Geometry: final body of the model. Coordinates: model frame, mm. Face numbers are marked on the shaded views. A direction names the side the tool comes from. Round coordinates to 2 decimals unless told otherwise and drop trailing zeros. Write each loop counter-clockwise with the first axis right and the second up, starting at its lowest first coordinate (ties: lowest second). Pieces come first, ordered by that corner, then holes. Notation, with made-up numbers: M -8.75,-6 L 32.25,-6 A24 ccw 32.25,15 Z; hole C 55.25,71 d3. An arc over 180 degrees is marked long. Answer as CSV lines item,"result". Start each with the question number.
Q1. Section query B-B on z = -1. Output: boundary loops of the cut face in (x, y), and give its area (3 significant figures).
Q2. Reachability of the marked faces 1 and 2 from +Z, -Z, +X, -X, +Y, -Y: full face, straight path, thin tool, end or side. Return the list, or none.
Q3. Mould query, pull axis Z, two halves, no side actions, for the marked faces 3, 4, 5 and 6. Classes: pulls with the +Z half, pulls with the -Z half, needs draft (parallel to the pull), parting line crosses it, or undercut.
Q4. Section query C-C on y = -6. Output: boundary loops of the cut face in (x, z).
Q5. Section query A-A on y = -19. Output: boundary loops of the cut face in (x, z), and give its area (3 significant figures).
Q6. Ray query, probe 1 along Y at (x, z) = (24.5, 4.25); probe 2 along Z at (x, y) = (15, -17); probe 3 along Z at (x, y) = (27, -32.5). Return the intervals inside material, ascending.
Q7. First-contact query: pin 1 (2 mm diameter, centred on x = 16, y = -18, fed in from -Z); pin 2 (3 mm diameter, centred on x = 18, z = 16, fed in from -Y); pin 3 (6 mm diameter, centred on x = 5, y = -34, fed in from +Z). Flat tips, straight axial feed; report the tip coordinate or a pass-through.
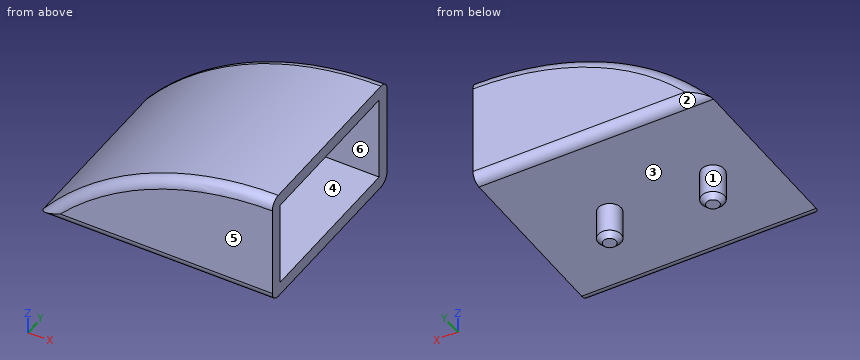
```python
from build123d import *

# Parameters (mm, degrees)
F1_DEPTH = 38
F2_T     = -2.6
F3_R     = 2
F5_DEPTH = 6.8
F6_SIZE  = 1


with BuildPart() as f1:
    # F0 (on Front) → F1 (new body)
    with BuildSketch(Plane.XZ):
        with BuildLine():
            ThreePointArc((46.1, 22), (20.5597866101, 16.218128967), (0, 0))
            Line((0, 0), (46.1, 0))
            Line((46.1, 0), (46.1, 22))
        make_face()
    extrude(amount=F1_DEPTH)

    # F2
    f2_openings = [f1.faces().sort_by_distance(p)[0] for p in [
        (46.1, -19, 11),
    ]]
    offset(amount=F2_T, openings=f2_openings)

    # F3
    f3_edges = [f1.edges().sort_by_distance(p)[0] for p in [
        (20.559787, -38, 16.218129),
        (20.559787, 0, 16.218129),
        (23.05, 0, 0),
        (23.05, -38, 0),
    ]]
    fillet(f3_edges, radius=F3_R)

    # F4 (on face) → F5 (join)
    with BuildSketch(Plane(origin=(0, 0, 0), x_dir=(1, 0, 0), z_dir=(0, 0, -1))):
        with BuildLine():
            Line((7.95, 19), (12.45, 19))
            ThreePointArc((12.45, 19), (10.2, 21.25), (7.95, 19))
        make_face()
        with BuildLine():
            ThreePointArc((7.95, 19), (10.2, 16.75), (12.45, 19))
            Line((12.45, 19), (7.95, 19))
        make_face()
        with BuildLine():
            ThreePointArc((32.75, 19), (30.5, 21.25), (28.25, 19))
            Line((28.25, 19), (32.75, 19))
        make_face()
        with BuildLine():
            Line((32.75, 19), (28.25, 19))
            ThreePointArc((28.25, 19), (30.5, 16.75), (32.75, 19))
        make_face()
    extrude(amount=F5_DEPTH)

    # F6
    f6_edges = [f1.edges().sort_by_distance(p)[0] for p in [
        (12.45, -19, -6.8),
        (32.75, -19, -6.8),
    ]]
    chamfer(f6_edges, length=F6_SIZE)


solid = f1.part
```
Entries:
1,outline,"C 10.2,-19 d4.5; C 30.5,-19 d4.5"
1,area,"31.8 mm^2"
2,face 1,"-Z"
2,face 2,"-Z, +X, -X, +Y"
3,face 3,"pulls with the -Z half"
3,face 4,"undercut"
3,face 5,"needs draft"
3,face 6,"undercut"
4,outline,"M 0,0 L 46.1,0 L 46.1,2.6 L 5.81,2.6 A56.7 cw 46.1,19.4 L 46.1,22 A59.3 ccw Z"
5,outline,"M 0,0 L 7.95,0 L 7.95,-5.8 L 8.95,-6.8 L 11.45,-6.8 L 12.45,-5.8 L 12.45,0 L 28.25,0 L 28.25,-5.8 L 29.25,-6.8 L 31.75,-6.8 L 32.75,-5.8 L 32.75,0 L 46.1,0 L 46.1,2.6 L 5.81,2.6 A56.7 cw 46.1,19.4 L 46.1,22 A59.3 ccw Z"
5,area,"299 mm^2"
6,probe 1,"y = -38 to -35.4, -2.6 to 0"
6,probe 2,"z = 0 to 2.6, 10.11 to 13.19"
6,probe 3,"z = 0 to 2.6, 16.09 to 18.84"
7,pin 1,"stops at z = 0"
7,pin 2,"stops at y = -37.37"
7,pin 3,"stops at z = 8.14"
